```python
from build123d import *

# Parameters (mm, degrees)
F0_W      = 465
F0_H      = 117
F1_DEPTH  = 60
F2_T      = -1
F3_W      = 182
F3_H      = 62
F3_W_2    = 20
F3_H_2    = 20
F3_R      = 1.5
F3_R_2    = 37.5
F3_W_3    = 104
F3_H_3    = 39
F4_DEPTH  = 25
F5_R      = 5
F6_R      = 2
F7_R      = 1.5
F8_DEPTH  = 500
F9_R      = 1.5
F10_DEPTH = 117.0010001
F11_DEPTH = 2


with BuildPart() as f1:
    # F0 (on Front) → F1 (new body)
    with BuildSketch(Plane.XZ):
        with Locations((-12.6529467106, 27.1878533959)):
            Rectangle(F0_W, F0_H)
    extrude(amount=F1_DEPTH)

    # F2
    f2_openings = [f1.faces().sort_by_distance(p)[0] for p in [
        (-12.652947, 0, 27.187853),
    ]]
    offset(amount=F2_T, openings=f2_openings)

    # F3 (on face) → F4 (cut)
    with BuildSketch(Plane.XZ.offset(60)):
        with Locations((-41.1529467106, 47.6878533959)):
            Rectangle(F3_W, F3_H)
        with Locations((76.8470532894, 68.6878533959)):
            Rectangle(F3_W_2, F3_H_2)
        Polygon((194.8470532894, 79.1878533959), (114.8470532894, 79.1878533959), (104.8470532894, 69.1878533959), (104.8470532894, -15.8121466041), (114.8470532894, -25.8121466041), (194.8470532894, -25.8121466041), (204.8470532894, -15.8121466041), (204.8470532894, 69.1878533959), align=None)
        with Locations((54.8470532894, 67.6878533959)):
            Circle(F3_R)
        with Locations((54.8470532894, 47.6878533959)):
            Circle(F3_R)
        with Locations((54.8470532894, 27.6878533959)):
            Circle(F3_R)
        with Locations((106.3470532894, 77.6878533959)):
            Circle(F3_R)
        Polygon((-87.1529467106, 8.1878533959), (-144.6529467106, 8.1878533959), (-152.1529467106, 0.6878533959), (-152.1529467106, -16.3121466041), (-144.6529467106, -23.8121466041), (-87.1529467106, -23.8121466041), (-79.6529467106, -16.3121466041), (-79.6529467106, 0.6878533959), align=None)
        with Locations((-193.6529467106, 20.1878533959)):
            Circle(F3_R_2)
        with Locations((-137.1529467106, 67.6878533959)):
            Circle(F3_R)
        with Locations((-137.1529467106, 47.6878533959)):
            Circle(F3_R)
        with Locations((-137.1529467106, 27.6878533959)):
            Circle(F3_R)
        with Locations((-223.6529467106, 50.1878533959)):
            Circle(F3_R)
        with Locations((-223.6529467106, -9.8121466041)):
            Circle(F3_R)
        with Locations((-163.6529467106, -9.8121466041)):
            Circle(F3_R)
        with Locations((-163.6529467106, 50.1878533959)):
            Circle(F3_R)
        with Locations((-57.1529467106, 8.6878533959)):
            Circle(F3_R)
        with Locations((52.8470532894, -24.3121466041)):
            Circle(F3_R)
        with Locations((-2.1529467106, -7.8121466041)):
            Rectangle(F3_W_3, F3_H_3)
        with Locations((-150.6529467106, 6.6878533959)):
            Circle(F3_R)
        with Locations((-81.1529467106, 6.6878533959)):
            Circle(F3_R)
        with Locations((-150.6529467106, -22.3121466041)):
            Circle(F3_R)
        with Locations((-81.1529467106, -22.3121466041)):
            Circle(F3_R)
        with Locations((203.3470532894, 77.6878533959)):
            Circle(F3_R)
        with Locations((106.3470532894, -24.3121466041)):
            Circle(F3_R)
        with Locations((203.3470532894, -24.3121466041)):
            Circle(F3_R)
    extrude(amount=-F4_DEPTH, mode=Mode.SUBTRACT)

    # F5
    f5_edges = [f1.edges().sort_by_distance(p)[0] for p in [
        (-245.152947, -30, 85.687853),
        (219.847053, -30, 85.687853),
        (219.847053, -30, -31.312147),
        (-245.152947, -30, -31.312147),
        (-244.152947, -29.5, 84.687853),
        (-244.152947, -29.5, -30.312147),
        (218.847053, -29.5, -30.312147),
        (218.847053, -29.5, 84.687853),
    ]]
    fillet(f5_edges, radius=F5_R)

    # F6
    f6_edges = [f1.edges().sort_by_distance(p)[0] for p in [
        (218.382587, -60, 84.223387),
        (-12.652947, -59, 84.687853),
    ]]
    fillet(f6_edges, radius=F6_R)

    # F7 (on face) → F8 (cut)
    with BuildSketch(Plane(origin=(-245.1529467106, 0, 0), x_dir=(0, -1, 0), z_dir=(-1, 0, 0))):
        with Locations((15, 47.1878533959)):
            Circle(F7_R)
        with Locations((15, 7.1878533959)):
            Circle(F7_R)
        with Locations((15, 27.1878533959)):
            Circle(F7_R)
    extrude(amount=-F8_DEPTH, mode=Mode.SUBTRACT)

    # F9 (on face) → F10 (cut, through all)
    with BuildSketch(Plane.XY.offset(85.6878533959)):
        with Locations((-201.1529467106, -35.5)):
            Circle(F9_R)
        with Locations((-104.6529467106, -35.5)):
            Circle(F9_R)
        with Locations((122.3470532894, -35.5)):
            Circle(F9_R)
        with Locations((181.3470532894, -35.5)):
            Circle(F9_R)
        with Locations((181.3470532894, -50.5)):
            Circle(F9_R)
    extrude(amount=-F10_DEPTH, mode=Mode.SUBTRACT)

    # F9 (on face) → F11 (cut)
    with BuildSketch(Plane.XY.offset(85.6878533959)):
        with Locations((76.8470532894, -35.5)):
            Circle(F9_R)
        with Locations((76.8470532894, -50.5)):
            Circle(F9_R)
    extrude(amount=-F11_DEPTH, mode=Mode.SUBTRACT)


solid = f1.part
```
Here's how the part is built. I have some questions about the finished solid (model axes, mm). A direction names the side the tool comes from. Coordinates: 2 decimals unless noted, no trailing zeros. Order: outer loops, then holes, each group sorted by start corner. A loop starts at its lowest first (then second) coordinate and runs counter-clockwise, first axis right, second up. Notation, with made-up numbers: M -30,-35 L -14,-35 A29 ccw -14,-3 Z; hole C 7.25,-37 d6. An arc over 180 degrees is marked long. Answer as a JSON object with one key per item and string values. Group by question number.
(1) I need wall thicknesses on probe 1 along Z at (x, y) = (-79, -12); probe 2 along X at (y, z) = (-52.5, -26); probe 3 along X at (y, z) = (-16.5, 17.5). Which ranges of each line are inside material? Lowest first, please.
(2) Which directions (+Z, -Z, +X, -X, +Y, -Y) give clear straight access to the entire face, cutting with the end or side of a thin tool? Please do faces 4 (the face through (-245.153, -29, 26)), 5 (the face through (-31, -59, 15)), 6 (the face through (-83.455, -59.507, -20.115)).
(3) Suppose I cut it at C-C, the plane y = -44. Please give me the cut outline in (x, z).
(4) Suppose I cut it at A-A, the plane x = 130. Please give me the cut outline in (y, z).
(5) For pin 1 (1.8 mm diameter, centred on x = 203.35, z = 77.69, fed in from -Y); pin 2 (0.8 mm diameter, centred on x = 0.5, y = -59.5, fed in from +Z), each with a flat end and sliding along its axis, tell me the tip position at first contact or that it passes through.
(6) Suppose I cut it at B-B, the plane x = -14. Please give me the cut outline in (y, z), then the cut area to 3 significant figures.
(7) If we mould it in two halves opening along Z, with no side actions, what happens to faces 1 (the face through (218.847, -28, 26)), 2 (the face through (-16, -29, -31.312)), 3 (the face through (219.847, -29, 26))? For each: released by +Z, released by -Z, zero draft, split by the parting line, or undercut.
Values found:
{
 "1": {"probe 1": "z = -31.31 to -30.31, 84.69 to 85.69", "probe 2": "x = -245.15 to -244.11, 218.8 to 219.85", "probe 3": "x = -245.15 to -244.15, 218.85 to 219.85"},
 "2": {"face 4": "+Z, -Z, -X, +Y, -Y", "face 5": "+Y", "face 6": "+Y, -Y"},
 "3": {"outline": "M -245.15,-26.31 A5 ccw -240.15,-31.31 L 214.85,-31.31 A5 ccw 219.85,-26.31 L 219.85,80.69 A5 ccw 214.85,85.69 L -240.15,85.69 A5 ccw -245.15,80.69 Z; hole M -244.15,-25.31 A5 ccw -239.15,-30.31 L 213.85,-30.31 A5 ccw 218.85,-25.31 L 218.85,79.69 A5 ccw 213.85,84.69 L -239.15,84.69 A5 ccw -244.15,79.69 Z"},
 "4": {"outline": "M -60,-29.31 A2 ccw -58,-31.31 L 0,-31.31 L 0,-30.31 L -57,-30.31 A2 cw -59,-28.31 L -59,-25.81 L -60,-25.81 Z; M -60,79.19 L -59,79.19 L -59,82.69 A2 cw -57,84.69 L 0,84.69 L 0,85.69 L -58,85.69 A2 ccw -60,83.69 Z"},
 "5": {"pin 1": "passes through", "pin 2": "stops at z = 85.36"},
 "6": {"outline": "M -60,-29.31 A2 ccw -58,-31.31 L 0,-31.31 L 0,-30.31 L -57,-30.31 A2 cw -59,-28.31 L -59,-27.31 L -60,-27.31 Z; M -60,11.69 L -59,11.69 L -59,16.69 L -60,16.69 Z; M -60,78.69 L -59,78.69 L -59,82.69 A2 cw -57,84.69 L 0,84.69 L 0,85.69 L -58,85.69 A2 ccw -60,83.69 Z", "area": "134 mm^2"},
 "7": {"face 1": "undercut", "face 2": "released by -Z", "face 3": "zero draft"}
}
